```python
from build123d import *

# Parameters (mm, degrees)
F0_W     = 167.259
F0_H     = 3.81
F0_W_2   = 5.588
F0_H_2   = 3.302
F1_DEPTH = 101.6


with BuildPart() as f1:
    # F0 (on Top) → F1 (new body)
    with BuildSketch(Plane.XY):
        with Locations((84.74498, 1.819537)):
            Rectangle(F0_W, F0_H)
        with Locations((4.16348, 1.819537)):
            Rectangle(F0_W_2, F0_H_2, mode=Mode.SUBTRACT)
        with Locations((10.13248, 1.819537)):
            Rectangle(F0_W_2, F0_H_2, mode=Mode.SUBTRACT)
        with Locations((16.10148, 1.819537)):
            Rectangle(F0_W_2, F0_H_2, mode=Mode.SUBTRACT)
        with Locations((22.07048, 1.819537)):
            Rectangle(F0_W_2, F0_H_2, mode=Mode.SUBTRACT)
        with Locations((28.03948, 1.819537)):
            Rectangle(F0_W_2, F0_H_2, mode=Mode.SUBTRACT)
        with Locations((34.00848, 1.819537)):
            Rectangle(F0_W_2, F0_H_2, mode=Mode.SUBTRACT)
        with Locations((39.97748, 1.819537)):
            Rectangle(F0_W_2, F0_H_2, mode=Mode.SUBTRACT)
        with Locations((45.94648, 1.819537)):
            Rectangle(F0_W_2, F0_H_2, mode=Mode.SUBTRACT)
        with Locations((51.91548, 1.819537)):
            Rectangle(F0_W_2, F0_H_2, mode=Mode.SUBTRACT)
        with Locations((57.88448, 1.819537)):
            Rectangle(F0_W_2, F0_H_2, mode=Mode.SUBTRACT)
        with Locations((63.85348, 1.819537)):
            Rectangle(F0_W_2, F0_H_2, mode=Mode.SUBTRACT)
        with Locations((69.82248, 1.819537)):
            Rectangle(F0_W_2, F0_H_2, mode=Mode.SUBTRACT)
        with Locations((75.79148, 1.819537)):
            Rectangle(F0_W_2, F0_H_2, mode=Mode.SUBTRACT)
        with Locations((81.76048, 1.819537)):
            Rectangle(F0_W_2, F0_H_2, mode=Mode.SUBTRACT)
        with Locations((87.72948, 1.819537)):
            Rectangle(F0_W_2, F0_H_2, mode=Mode.SUBTRACT)
        with Locations((93.69848, 1.819537)):
            Rectangle(F0_W_2, F0_H_2, mode=Mode.SUBTRACT)
        with Locations((99.66748, 1.819537)):
            Rectangle(F0_W_2, F0_H_2, mode=Mode.SUBTRACT)
        with Locations((105.63648, 1.819537)):
            Rectangle(F0_W_2, F0_H_2, mode=Mode.SUBTRACT)
        with Locations((111.60548, 1.819537)):
            Rectangle(F0_W_2, F0_H_2, mode=Mode.SUBTRACT)
        with Locations((117.57448, 1.819537)):
            Rectangle(F0_W_2, F0_H_2, mode=Mode.SUBTRACT)
        with Locations((123.54348, 1.819537)):
            Rectangle(F0_W_2, F0_H_2, mode=Mode.SUBTRACT)
        with Locations((129.51248, 1.819537)):
            Rectangle(F0_W_2, F0_H_2, mode=Mode.SUBTRACT)
        with Locations((135.48148, 1.819537)):
            Rectangle(F0_W_2, F0_H_2, mode=Mode.SUBTRACT)
        with Locations((141.45048, 1.819537)):
            Rectangle(F0_W_2, F0_H_2, mode=Mode.SUBTRACT)
        with Locations((147.41948, 1.819537)):
            Rectangle(F0_W_2, F0_H_2, mode=Mode.SUBTRACT)
        with Locations((153.38848, 1.819537)):
            Rectangle(F0_W_2, F0_H_2, mode=Mode.SUBTRACT)
        with Locations((159.35748, 1.819537)):
            Rectangle(F0_W_2, F0_H_2, mode=Mode.SUBTRACT)
        with Locations((165.32648, 1.819537)):
            Rectangle(F0_W_2, F0_H_2, mode=Mode.SUBTRACT)
    extrude(amount=F1_DEPTH)


solid = f1.part
```
Geometry: final body of the model. Coordinates: model frame, mm. Give positions to 0.01 mm unless a question says otherwise; leave off trailing zeros. Write each loop counter-clockwise with the first axis right and the second up, starting at its lowest first coordinate (ties: lowest second). Pieces come first, ordered by that corner, then holes.
1. Line query: probe 1 along Y at (x, z) = (8.5, 59). Output: solid intervals per line, ascending.
2. Section query A-A, the plane x = 69. Return loops of the section in (y, z).
3. Section query B-B, the plane z = 83.5. Count the separate pieces of the cut face and the enclosed holes in it, then the cut area to 3 significant figures.
Computed:
1. probe 1: y = -0.09 to 0.17, 3.47 to 3.72
2. outline: (-0.09, 0) - (0.17, 0) - (0.17, 101.6) - (-0.09, 101.6) - close; (3.47, 0) - (3.72, 0) - (3.72, 101.6) - (3.47, 101.6) - close
3. separate pieces: 1
3. enclosed holes: 28
3. area: 121 mm2
